Geometry: final body of the model. Coordinates: model frame, mm. Give positions to 0.01 mm unless a question says otherwise; leave off trailing zeros. Loops run counter-clockwise (first coordinate to the right, second up) from the corner with the lowest first, then second, coordinate; pieces in that order, holes last. Notation, with made-up numbers: M 46,-20.5 L 51,-20.5 A14 ccw 51,-8.5 Z; hole C -19,48 d10. An arc over 180 degrees is marked long. Put each result on its own line as item: value.
```python
from build123d import *

# Parameters (mm, degrees)
SKETCH1_W           = 680
SKETCH1_H           = 680
SKETCH1_W_2         = 600
SKETCH1_H_2         = 600
BOSS_EXTRUDE1_DEPTH = 40
SKETCH2_W           = 20
SKETCH2_H           = 20
CUT_EXTRUDE2_DEPTH  = 30
SKETCH3_R           = 2.5
CUT_EXTRUDE3_DEPTH  = 40
CUT_EXTRUDE4_START  = -40
SKETCH4_R           = 2.5
CUT_EXTRUDE4_DEPTH  = 40


with BuildPart() as part:
    # Sketch1 → Boss-Extrude1 (new body)
    with BuildSketch(Plane(origin=(0, 0, 0), x_dir=(1, 0, 0), z_dir=(0, 1, 0))):
        Rectangle(SKETCH1_W, SKETCH1_H)
        Rectangle(SKETCH1_W_2, SKETCH1_H_2, mode=Mode.SUBTRACT)
    extrude(amount=BOSS_EXTRUDE1_DEPTH)

    # Sketch2 → Cut-Extrude2 (cut)
    with BuildSketch(Plane(origin=(0, 40, 0), x_dir=(1, 0, 0), z_dir=(0, 1, 0))):
        with Locations((-320.027392849, 320)):
            Rectangle(SKETCH2_W, SKETCH2_H)
        with Locations((319.972607151, 320)):
            Rectangle(SKETCH2_W, SKETCH2_H)
        with Locations((319.972607151, -320)):
            Rectangle(SKETCH2_W, SKETCH2_H)
        with Locations((-320.027392849, -320)):
            Rectangle(SKETCH2_W, SKETCH2_H)
    extrude(amount=-CUT_EXTRUDE2_DEPTH, mode=Mode.SUBTRACT)

    # Sketch3 → Cut-Extrude3 (cut)
    with BuildSketch(Plane(origin=(0, 0, -340), x_dir=(-1, 0, 0), z_dir=(0, 0, -1))):
        with Locations((320, 25)):
            Circle(SKETCH3_R)
        with Locations((-320, 25)):
            Circle(SKETCH3_R)
    extrude(amount=-CUT_EXTRUDE3_DEPTH, mode=Mode.SUBTRACT)

    # Sketch4 → Cut-Extrude4 (cut)
    with BuildSketch(Plane.XY.offset(340).offset(CUT_EXTRUDE4_START)):
        with Locations(Location((-320, 25, 0), (0, 0, 180))):
            Circle(SKETCH4_R)
        with Locations(Location((320, 25, 0), (0, 0, 180))):
            Circle(SKETCH4_R)
    extrude(amount=CUT_EXTRUDE4_DEPTH, mode=Mode.SUBTRACT)


solid = part.part
```
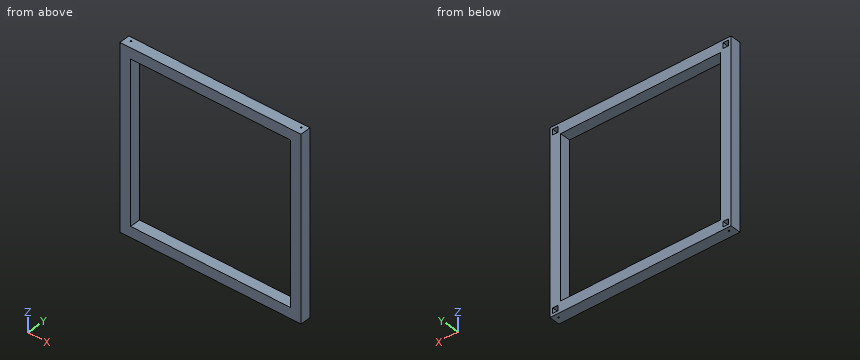
Item 1: Section C-C on x = 2. Output: boundary loops of the cut face in (y, z), then the cut area to 3 significant figures.
Output values:
outline: M 0,-340 L 40,-340 L 40,-300 L 0,-300 Z; M 0,300 L 40,300 L 40,340 L 0,340 Z
area: 3,200 mm²
Item 2: Pin query (flat end, axial travel): pin 1 Ø1.5 at (x, y) = (320, 25.5) entering from -Z; pin 2 Ø6 at (x, z) = (-318.5, 317.5) entering from +Y; pin 3 Ø4 at (x, y) = (-320, 25) entering from +Z. Return the tip coordinate at first contact, or that it passes through.
Output values:
pin 1: z = -300
pin 2: y = 10
pin 3: z = 300
Item 3: Line query: probe 1 along X at (y, z) = (25, 332); probe 2 along Z at (x, y) = (-7.5, 27); probe 3 along Y at (x, z) = (-320, -333.25). Output: solid intervals per line, ascending. Write a range as [from, to].
Output values:
probe 1: [-340, -322.5], [-317.5, 317.5], [322.5, 340]
probe 2: [-340, -300], [300, 340]
probe 3: [0, 22.5], [27.5, 40]
Item 4: Section A-A on y = 33.5. Output: boundary loops of the cut face in (x, z), then the cut area to 3 significant figures.
Output values:
outline: M -340,-340 L 340,-340 L 340,340 L -340,340 Z; hole M -330.03,-330 L -310.03,-330 L -310.03,-310 L -330.03,-310 Z; hole M -330.03,310 L -310.03,310 L -310.03,330 L -330.03,330 Z; hole M -300,-300 L 300,-300 L 300,300 L -300,300 Z; hole M 309.97,-330 L 329.97,-330 L 329.97,-310 L 309.97,-310 Z; hole M 309.97,310 L 329.97,310 L 329.97,330 L 309.97,330 Z
area: 101,000 mm²
Item 5: Section B-B on z = 189. Output: boundary loops of the cut face in (x, y), then the cut area to 3 significant figures.
Output values:
outline: M -340,0 L -300,0 L -300,40 L -340,40 Z; M 300,0 L 340,0 L 340,40 L 300,40 Z
area: 3,200 mm²
